Part model, mm, in its own coordinate system. A direction names the side the tool comes from. Round coordinates to 2 decimals unless told otherwise and drop trailing zeros. Loops run counter-clockwise (first coordinate to the right, second up) from the corner with the lowest first, then second, coordinate; pieces in that order, holes last.
from build123d import *

# Parameters (mm, degrees)
ESTRUSIONE_ESTRUSIONE1_DEPTH = 8.5
RACCORDO1_R                  = 10
SCHIZZO2_R                   = 40
ESTRUSIONE_ESTRUSIONE2_DEPTH = 20
RACCORDO2_START              = 8.5
RACCORDO2_DEPTH              = 5.0000001
SCHIZZO3_R                   = 1.5
TAGLIO_ESTRUSIONE1_DEPTH     = 20
SCHIZZO4_R                   = 36
TAGLIO_ESTRUSIONE2_DEPTH     = 21


with BuildPart() as part:
    # Schizzo1 → Estrusione-Estrusione1 (new body)
    with BuildSketch(Plane.XY):
        with BuildLine():
            ThreePointArc((-20.628430767, -34.270509831), (0, -40), (20.628430767, -34.270509831))
            ThreePointArc((20.628430767, -34.270509831), (51.961524227, -30), (39.993347498, -0.729490169))
            ThreePointArc((39.993347498, -0.729490169), (34.641016151, 20), (19.364916731, 35))
            ThreePointArc((19.364916731, 35), (0, 60), (-19.364916731, 35))
            ThreePointArc((-19.364916731, 35), (-34.641016151, 20), (-39.993347498, -0.729490169))
            ThreePointArc((-39.993347498, -0.729490169), (-51.961524227, -30), (-20.628430767, -34.270509831))
        make_face()
    extrude(amount=ESTRUSIONE_ESTRUSIONE1_DEPTH)

    # Raccordo1
    raccordo1_edges = [part.edges().sort_by_distance(p)[0] for p in [
        (39.993347498, -0.729490169, 4.25),
        (20.628430767, -34.270509831, 4.25),
        (-20.628430767, -34.270509831, 4.25),
        (-39.993347498, -0.729490169, 4.25),
        (-19.364916731, 35, 4.25),
        (19.364916731, 35, 4.25),
    ]]
    fillet(raccordo1_edges, radius=RACCORDO1_R)

    # Schizzo2 → Estrusione-Estrusione2 (add)
    with BuildSketch(Plane.XY.offset(8.5)):
        with Locations(Location((0, 0, 0), (0, 0, 173.130102354))):
            Circle(SCHIZZO2_R)
    extrude(amount=ESTRUSIONE_ESTRUSIONE2_DEPTH)

    # Raccordo2: read off the stored shape, not the designer's step
    # Raccordo2 outline → Raccordo2 (add)
    with BuildSketch(Plane.XY.offset(RACCORDO2_START)):
        with BuildLine():
            ThreePointArc((-20, 40), (-21.05572809, 35.527864045), (-24, 32))
            ThreePointArc((-24, 32), (0, 40), (24, 32))
            ThreePointArc((24, 32), (21.05572809, 35.527864045), (20, 40))
            ThreePointArc((20, 40), (0, 60), (-20, 40))
        make_face()
        with BuildLine():
            ThreePointArc((-15.712812921, -36.784609691), (-34.641016151, -20), (-39.712812921, 4.784609691))
            ThreePointArc((-39.712812921, 4.784609691), (-41.29589685, 0.470863399), (-44.641016151, -2.679491924))
            ThreePointArc((-44.641016151, -2.679491924), (-51.961524227, -30), (-24.641016151, -37.320508076))
            ThreePointArc((-24.641016151, -37.320508076), (-20.24016876, -35.998727444), (-15.712812921, -36.784609691))
        make_face()
        with BuildLine():
            ThreePointArc((44.641016151, -2.679491924), (41.29589685, 0.470863399), (39.712812921, 4.784609691))
            ThreePointArc((39.712812921, 4.784609691), (34.641016151, -20), (15.712812921, -36.784609691))
            ThreePointArc((15.712812921, -36.784609691), (20.24016876, -35.998727444), (24.641016151, -37.320508076))
            ThreePointArc((24.641016151, -37.320508076), (51.961524227, -30), (44.641016151, -2.679491924))
        make_face()
    extrude(amount=RACCORDO2_DEPTH)

    # Raccordo2 2 outline → Raccordo2 2 (revolve, cut)
    with BuildSketch(Plane.XZ):
        with BuildLine():
            ThreePointArc((40, 13.5), (41.464466094, 9.964466094), (45, 8.5))
            Line((45, 8.5), (60, 8.5))
            Line((60, 8.5), (60, 13.5000001))
            Line((60, 13.5000001), (40, 13.5))
        make_face()
    revolve(axis=Axis((0, 0, 0), (0, 0, 1)), mode=Mode.SUBTRACT)

    # Schizzo3 → Taglio-Estrusione1 (cut)
    with BuildSketch(Plane.XY.offset(8.5)):
        with Locations((0, 52.5)):
            Circle(SCHIZZO3_R)
        with Locations((-45.466333699, -26.25)):
            Circle(SCHIZZO3_R)
        with Locations((45.466333699, -26.25)):
            Circle(SCHIZZO3_R)
    extrude(amount=-TAGLIO_ESTRUSIONE1_DEPTH, mode=Mode.SUBTRACT)

    # Schizzo4 → Taglio-Estrusione2 (cut)
    with BuildSketch(Plane.XY.offset(28.5)):
        Circle(SCHIZZO4_R)
    extrude(amount=-TAGLIO_ESTRUSIONE2_DEPTH, mode=Mode.SUBTRACT)


solid = part.part
1) Tool access for faces 1 (the face through (-40.32, 2.36, 9.85)), 2 (the face through (-43, -25, 8.5)), 3 (the face through (-4.686, 35.694, 18.147)): list every direction of +Z, -Z, +X, -X, +Y, -Y with a clear straight run to the whole face (end or side of a thin tool).
Values:
face 1: +Z, -Z, -X, +Y
face 2: +Z, -X, -Y
face 3: +Z
2) Mould opens along X. For faces 4 (the face through (43, -25, 8.5)), 5 (the face through (-22, 34, 10)), 6 (the face through (-18.25, -36.08, 9.85)), 7 (the face through (-1, 1, 7.5)) say: released by +X, released by -X, zero draft, split by the parting line, or undercut.
Values:
face 4: zero draft
face 5: released by -X
face 6: undercut
face 7: undercut
3) Slice it at B-B, the plane z = 12.25. Give the cut face in (x, y), then the cut area to 3 significant figures.
Values:
outline: (-40.03, 3.22) arc R40.16 ccw to (-17.23, -36.28) arc R10 cw to (-15.71, -36.78) arc R40 ccw to (15.71, -36.78) arc R10 cw to (17.23, -36.28) arc R40.16 ccw to (40.03, 3.22) arc R10 cw to (39.71, 4.78) arc R40 ccw to (24, 32) arc R10 cw to (22.8, 33.06) arc R40.16 ccw to (-22.8, 33.06) arc R10 cw to (-24, 32) arc R40 ccw to (-39.71, 4.78) arc R10 cw to start; hole circle Ø72 at (0, 0)
area: 979 mm2
4) Drop flat-ended pins along their axis: pin 1 Ø3 at (x, z) = (-10.5, 8.5) entering from +Y; pin 2 Ø10 at (x, y) = (6, 49) entering from +Z; pin 3 Ø2 at (y, z) = (25, 14.5) entering from -X. Give the stop position or say it passes through.
Values:
pin 1: stops at y = 57.86
pin 2: stops at z = 8.54
pin 3: stops at x = -32
5) Slice it at D-D, the plane z = 24.75. Give the cut face in (x, y).
Values:
outline: circle Ø80 at (0, 0); hole circle Ø72 at (0, 0)
6) Slice it at A-A, the plane x = 0. Give the cut face in (y, z).
Values:
outline: (-40, 0) - (51, 0) - (51, 8.5) - (45, 8.5) arc R5 cw to (40, 13.5) - (40, 28.5) - (36, 28.5) - (36, 7.5) - (-36, 7.5) - (-36, 28.5) - (-40, 28.5) - close; (54, 0) - (60, 0) - (60, 8.5) - (54, 8.5) - close
7) Slice it at C-C, the plane y = -26.25. Give the number of separate pieces and of enclosed holes in the cut face, then the cut area to 3 significant figures.
Values:
separate pieces: 3
enclosed holes: 0
area: 1,050 mm2
8) Wall check: line 1 along Y through (x, z) = (-0.5, 19.5); line 2 along Z through (x, y) = (-16.5, 8.5); line 3 along Y through (x, z) = (-28.5, 25.5). Give the ranges that are in metal, low to high.
Values:
line 1: y = -40 to -36, 36 to 40
line 2: z = 0 to 7.5
line 3: y = -28.07 to -21.99, 21.99 to 28.07
